```python
from build123d import *

# Parameters (mm, degrees)
F0_R     = 0.5
F1_DEPTH = 1
F2_DEPTH = 13.23
F3_R     = 1.8
F4_DEPTH = 1
F6_DEPTH = 1


with BuildPart() as f1:
    # F0 (on Top) → F1 (new body)
    with BuildSketch(Plane.XY):
        with BuildLine():
            ThreePointArc((-17.84133, -20.107526), (-17.255543, -21.521739), (-15.84133, -22.107526))
            Line((-15.84133, -22.107526), (15.15867, -22.107526))
            ThreePointArc((15.15867, -22.107526), (16.572884, -21.521739), (17.15867, -20.107526))
            Line((17.15867, -20.107526), (17.15867, 25.892474))
            ThreePointArc((17.15867, 25.892474), (16.572884, 27.306688), (15.15867, 27.892474))
            Line((15.15867, 27.892474), (-15.84133, 27.892474))
            ThreePointArc((-15.84133, 27.892474), (-17.255543, 27.306688), (-17.84133, 25.892474))
            Line((-17.84133, 25.892474), (-17.84133, -20.107526))
        make_face()
        with Locations((-15.84133, -20.107526)):
            Circle(F0_R, mode=Mode.SUBTRACT)
        with Locations((15.15867, -20.107526)):
            Circle(F0_R, mode=Mode.SUBTRACT)
        with Locations((-15.84133, 25.892474)):
            Circle(F0_R, mode=Mode.SUBTRACT)
        with Locations((15.15867, 25.892474)):
            Circle(F0_R, mode=Mode.SUBTRACT)
    extrude(amount=F1_DEPTH)

    # F0 (on Top) → F2 (join)
    with BuildSketch(Plane.XY):
        with BuildLine():
            Line((15.15867, 28.892474), (-15.84133, 28.892474))
            ThreePointArc((-15.84133, 28.892474), (-17.96265, 28.013795), (-18.84133, 25.892474))
            Line((-18.84133, 25.892474), (-18.84133, -20.107526))
            ThreePointArc((-18.84133, -20.107526), (-17.96265, -22.228846), (-15.84133, -23.107526))
            Line((-15.84133, -23.107526), (15.15867, -23.107526))
            ThreePointArc((15.15867, -23.107526), (17.279991, -22.228846), (18.15867, -20.107526))
            Line((18.15867, -20.107526), (18.15867, 25.892474))
            ThreePointArc((18.15867, 25.892474), (17.279991, 28.013795), (15.15867, 28.892474))
        make_face()
        with BuildLine():
            Line((15.15867, -22.107526), (-15.84133, -22.107526))
            ThreePointArc((-15.84133, -22.107526), (-17.255543, -21.521739), (-17.84133, -20.107526))
            Line((-17.84133, -20.107526), (-17.84133, 25.892474))
            ThreePointArc((-17.84133, 25.892474), (-17.255543, 27.306688), (-15.84133, 27.892474))
            Line((-15.84133, 27.892474), (15.15867, 27.892474))
            ThreePointArc((15.15867, 27.892474), (16.572884, 27.306688), (17.15867, 25.892474))
            Line((17.15867, 25.892474), (17.15867, -20.107526))
            ThreePointArc((17.15867, -20.107526), (16.572884, -21.521739), (15.15867, -22.107526))
        make_face(mode=Mode.SUBTRACT)
    extrude(amount=F2_DEPTH)

    # F3 (on face) → F4 (cut)
    with BuildSketch(Plane(origin=(0, 0, 0), x_dir=(1, 0, 0), z_dir=(0, 0, -1))):
        with Locations((-7.26933, -22.408474)):
            Circle(F3_R)
        with Locations((7.54767, -22.408474)):
            Circle(F3_R)
    extrude(amount=-F4_DEPTH, mode=Mode.SUBTRACT)

    # F5 (on face) → F6 (join)
    with BuildSketch(Plane.XY.offset(13.23)):
        with BuildLine():
            Line((15.15867, 30.892474), (-15.84133, 30.892474))
            ThreePointArc((-15.84133, 30.892474), (-19.376864, 29.428008), (-20.84133, 25.892474))
            Line((-20.84133, 25.892474), (-20.84133, -20.107526))
            ThreePointArc((-20.84133, -20.107526), (-19.376864, -23.64306), (-15.84133, -25.107526))
            Line((-15.84133, -25.107526), (15.15867, -25.107526))
            ThreePointArc((15.15867, -25.107526), (18.694204, -23.64306), (20.15867, -20.107526))
            Line((20.15867, -20.107526), (20.15867, 25.892474))
            ThreePointArc((20.15867, 25.892474), (18.694204, 29.428008), (15.15867, 30.892474))
        make_face()
        with BuildLine():
            ThreePointArc((15.15867, 28.892474), (17.279991, 28.013795), (18.15867, 25.892474))
            Line((18.15867, 25.892474), (18.15867, -20.107526))
            ThreePointArc((18.15867, -20.107526), (17.279991, -22.228846), (15.15867, -23.107526))
            Line((15.15867, -23.107526), (-15.84133, -23.107526))
            ThreePointArc((-15.84133, -23.107526), (-17.96265, -22.228846), (-18.84133, -20.107526))
            Line((-18.84133, -20.107526), (-18.84133, 25.892474))
            ThreePointArc((-18.84133, 25.892474), (-17.96265, 28.013795), (-15.84133, 28.892474))
            Line((-15.84133, 28.892474), (15.15867, 28.892474))
        make_face(mode=Mode.SUBTRACT)
    extrude(amount=-F6_DEPTH)


solid = f1.part
```
Geometry: final body of the model. Coordinates: model frame, mm. A direction names the side the tool comes from. Round coordinates to 2 decimals unless told otherwise and drop trailing zeros. Write each loop counter-clockwise with the first axis right and the second up, starting at its lowest first coordinate (ties: lowest second). Pieces come first, ordered by that corner, then holes.
Item 1: Pin query (flat end, axial travel): P1, Ø1, axis at x = -6.5, z = 9, coming from the -Y side; P2, Ø3.5, axis at y = 0.5, z = 7.5, coming from the -X side; P3, Ø6, axis at y = -1, z = 5.5, coming from the +X side. Return the tip coordinate at first contact, or that it passes through.
Item 2: Set-up query: faces 1 (the face through (-20, 3, 12.23)), 2 (the face through (-17.939, 28.037, 6.029)), 3 (the face through (17.303, 27.99, 6.029)), 4 (the face through (-1, 27.892, 7)). Return all of +Z, -Z, +X, -X, +Y, -Y with unobstructed straight access to the full face (end or side cutting, diameter ignored); none if empty.
Item 3: Section query A-A (z = 9.5). Return loops of the section in (x, y), plus the area to 3 significant figures.
Item 4: Section query C-C (y = 6.5). Return loops of the section in (x, z).
Item 5: Mould query, pull axis X, two halves, no side actions, for faces 5 (the face through (-19.42, -23.6, 12.74)), 6 (the face through (16.588, -21.506, 7.029)), 7 (the face through (-1, -23.108, 6)). Classes: +X half, -X half, draft (parallel to the pull), parting line (faces both ways), or undercut.
Item 6: Material intervals for L1, parallel to Y at x = -16, z = 3.25; L2, parallel to X at y = 21, z = 2; L3, parallel to Y at x = 10, z = 12.5, sorted ascending.
Item 7: Section query B-B (x = 4.5). Return loops of the section in (y, z), plus the area to 3 significant figures.
Completed:
1. P1: stops at y = -23.11
1. P2: stops at x = -18.84
1. P3: stops at x = 18.16
2. face 1: -Z
2. face 2: -Z, -X, +Y
2. face 3: -Z, +X, +Y
2. face 4: +Z
3. outline: (-18.84, -20.11) arc R3 ccw to (-15.84, -23.11) - (15.16, -23.11) arc R3 ccw to (18.16, -20.11) - (18.16, 25.89) arc R3 ccw to (15.16, 28.89) - (-15.84, 28.89) arc R3 ccw to (-18.84, 25.89) - close; hole (-17.84, -20.11) arc R2 ccw to (-15.84, -22.11) - (15.16, -22.11) arc R2 ccw to (17.16, -20.11) - (17.16, 25.89) arc R2 ccw to (15.16, 27.89) - (-15.84, 27.89) arc R2 ccw to (-17.84, 25.89) - close
3. area: 170 mm2
4. outline: (-20.84, 12.23) - (-18.84, 12.23) - (-18.84, 0) - (18.16, 0) - (18.16, 12.23) - (20.16, 12.23) - (20.16, 13.23) - (17.16, 13.23) - (17.16, 1) - (-17.84, 1) - (-17.84, 13.23) - (-20.84, 13.23) - close
5. face 5: -X half
5. face 6: undercut
5. face 7: draft
6. L1: y = -23.1 to -22.1, 27.89 to 28.89
6. L2: x = -18.84 to -17.84, 17.16 to 18.16
6. L3: y = -25.11 to -22.11, 27.89 to 30.89
7. outline: (-25.11, 12.23) - (-23.11, 12.23) - (-23.11, 0) - (28.89, 0) - (28.89, 12.23) - (30.89, 12.23) - (30.89, 13.23) - (27.89, 13.23) - (27.89, 1) - (-22.11, 1) - (-22.11, 13.23) - (-25.11, 13.23) - close
7. area: 80.5 mm2
